The listing builds one solid part. Answer for the finished solid, in the listing's coordinates (mm). Give positions to 0.01 mm unless a question says otherwise; leave off trailing zeros. Write each loop counter-clockwise with the first axis right and the second up, starting at its lowest first coordinate (ties: lowest second). Pieces come first, ordered by that corner, then holes.
```python
from build123d import *

# Parameters (mm, degrees)
F0_R     = 16.418587
F0_R_2   = 6.310263
F1_DEPTH = 25.4
F2_R     = 5.08
F3_R     = 2.54


with BuildPart() as f1:
    # F0 (on Front) → F1 (new body)
    with BuildSketch(Plane.XZ):
        with BuildLine():
            ThreePointArc((-57.30524, -24.439051), (-43.965646, -15.3196), (-38.825702, 0))
            ThreePointArc((-38.825702, 0), (-44.145238, 15.55426), (-57.875702, 24.593444))
            ThreePointArc((-57.875702, 24.593444), (-89.623983, -0.295493), (-57.30524, -24.439051))
        make_face()
        with Locations((-64.225702, 0)):
            Circle(F0_R, mode=Mode.SUBTRACT)
        with BuildLine():
            ThreePointArc((-57.875702, 24.593444), (-44.145238, 15.55426), (-38.825702, 0))
            ThreePointArc((-38.825702, 0), (-43.965646, -15.3196), (-57.30524, -24.439051))
            Line((-57.30524, -24.439051), (-15.338253, -12.555164))
            ThreePointArc((-15.338253, -12.555164), (-25.867667, 2.547056), (-10.250702, 12.296722))
            Line((-10.250702, 12.296722), (-57.875702, 24.593444))
        make_face()
        with BuildLine():
            ThreePointArc((-0.725702, 0), (-3.38547, 7.77713), (-10.250702, 12.296722))
            ThreePointArc((-10.250702, 12.296722), (-25.867667, 2.547056), (-15.338253, -12.555164))
            ThreePointArc((-15.338253, -12.555164), (-5.149211, -9.632741), (-0.725702, 0))
        make_face()
        with Locations((-13.425702, 0)):
            Circle(F0_R_2, mode=Mode.SUBTRACT)
    extrude(amount=F1_DEPTH)

    # F2
    f2_edges = [f1.edges().sort_by_distance(p)[0] for p in [
        (-80.644288, -25.4, 0),
        (-7.115439, -12.7, 0),
        (-19.735965, 0, 0),
        (-19.735965, -25.4, 0),
    ]]
    fillet(f2_edges, radius=F2_R)

    # F3
    f3_edges = [f1.edges().sort_by_distance(p)[0] for p in [
        (-80.644288, 0, 0),
    ]]
    fillet(f3_edges, radius=F3_R)


solid = f1.part
```
Item 1: Determine the mould class of faces 1 (the face through (-77.255, -11.306, -9.99)), 2 (the face through (-33.73, -12.52, 18.36)), 3 (the face through (-89.623, -12.522, 0.357)), 4 (the face through (-46, 0, 6)) for opening direction X: pulls with the +X half, pulls with the -X half, needs draft (parallel to the pull), parting line crosses it, or undercut.
Conclusion:
face 1: undercut
face 2: pulls with the +X half
face 3: parting line crosses it
face 4: needs draft
Item 2: A cutting plane is placed at D-D, the plane y = -1.5. Give the vertices of the cut face in (x, z).
Conclusion:
outline: (-57.88, 24.59) arc R25.4 ccw (long way) to (-57.31, -24.44) - (-15.34, -12.56) arc R12.7 ccw to (-0.73, 0) arc R12.7 ccw to (-10.25, 12.3) - close; hole circle Ø33.28 at (-64.23, 0); hole circle Ø15.57 at (-13.43, 0)
Item 3: A cutting plane is placed at A-A, the plane y = -18.25. Give the vertices of the cut face in (x, z).
Conclusion:
outline: (-57.88, 24.59) arc R25.4 ccw (long way) to (-57.31, -24.44) - (-15.34, -12.56) arc R12.7 ccw to (-0.73, 0) arc R12.7 ccw to (-10.25, 12.3) - close; hole circle Ø32.84 at (-64.23, 0); hole circle Ø12.62 at (-13.43, 0)
Item 4: A cutting plane is placed at C-C, the plane x = -41.5. Give the vertices of the cut face in (y, z), plus the area to 3 significant figures.
Conclusion:
outline: (-25.4, -19.96) - (0, -19.96) - (0, 20.37) - (-25.4, 20.37) - close
area: 1,020 mm2
Item 5: A cutting plane is placed at B-B, the plane z = 3. Count the separate pieces of the cut face and the enclosed holes in it, plus the area to 3 significant figures.
Conclusion:
separate pieces: 3
enclosed holes: 0
area: 1,100 mm2
Item 6: Consider probe 1 along X at (y, z) = (-8.5, -4); probe 2 along X at (y, z) = (-16.25, 3.5); probe 3 along Z at (x, y) = (-12, -14.5). Determine where each line is inside the solid, lowest interval first.
Conclusion:
probe 1: x = -89.31 to -80.15, -48.3 to -18.31, -8.55 to -1.37
probe 2: x = -89.38 to -80.27, -48.18 to -18.68, -8.18 to -1.22
probe 3: z = -12.62 to -6.15, 6.15 to 12.75
Item 7: Each of these flat-tipped pins is pushed along its axis until it touches: P1, Ø5, axis at y = -14.5, z = -13, coming from the -X side; P2, Ø5, axis at y = -19.5, z = 4, coming from the -X side; P3, Ø4, axis at x = -59, y = -10.5, coming from the +Z side. Where does it stop, or does it pass through?
Conclusion:
P1: stops at x = -87.35
P2: stops at x = -89.58
P3: stops at z = 25.19
